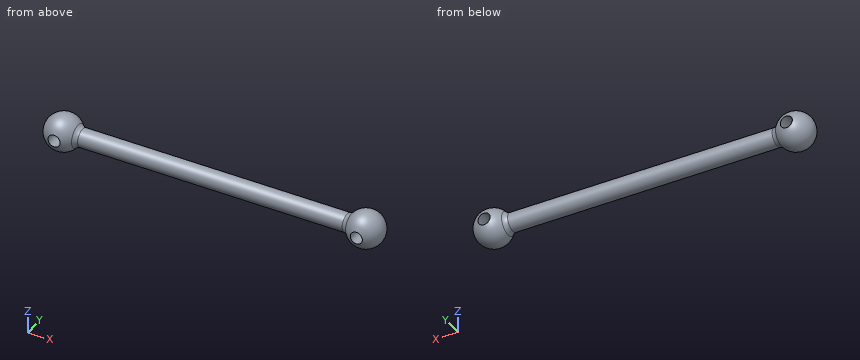
```python
from build123d import *

# Parameters (mm, degrees)
SKETCH1_W          = 23
SKETCH1_H          = 1.5
SKETCH2_R          = 1
CUT_EXTRUDE1_DEPTH = 29.792360098
FILLET1_R          = 1
FILLET2_R          = 1


with BuildPart() as part:
    # Sketch1 → Revolve2 (revolve)
    with BuildSketch(Plane.XY, mode=Mode.PRIVATE) as revolve2_sk:
        with BuildLine():
            Line((23, 1.5), (23, 0))
            Line((23, 0), (28, 0))
            ThreePointArc((28, 0), (25.776457135, 2.897777479), (22.401923789, 1.5))
            Line((22.401923789, 1.5), (23, 1.5))
        make_face()
        with Locations((11.5, 0.75)):
            Rectangle(SKETCH1_W, SKETCH1_H)
    revolve2 = revolve(revolve2_sk.sketch.rotate(Axis((0, 0, 0), (1, 0, 0)), 90), axis=Axis((0, 0, 0), (1, 0, 0)))

    # Sketch2 → Cut-Extrude1 (cut, through all)
    with BuildSketch(Plane(origin=(0, 3, 0), x_dir=(1, 0, 0), z_dir=(0, 1, 0))):
        with Locations(Location((25, 0, 0), (0, 0, 270))):
            Circle(SKETCH2_R)
    cut_extrude1 = extrude(amount=-CUT_EXTRUDE1_DEPTH, mode=Mode.SUBTRACT)

    # Mirror1: Revolve2, Cut-Extrude1 across plane
    add(revolve2.mirror(Plane.ZY))
    add(cut_extrude1.mirror(Plane.ZY), mode=Mode.SUBTRACT)

    # Fillet1
    fillet1_edges = [part.edges().sort_by_distance(p)[0] for p in [
        (22.401923789, 0, -1.5),
    ]]
    fillet(fillet1_edges, radius=FILLET1_R)

    # Fillet2
    fillet2_edges = [part.edges().sort_by_distance(p)[0] for p in [
        (-22.401923789, 0, -1.5),
    ]]
    fillet(fillet2_edges, radius=FILLET2_R)


solid = part.part
```
Work out the finished part from the listing and answer in its coordinate system (mm). Give positions to 0.01 mm unless a question says otherwise; leave off trailing zeros. Order: outer loops, then holes, each group sorted by start corner. A loop starts at its lowest first (then second) coordinate and runs counter-clockwise, first axis right, second up. Notation, with made-up numbers: (46.5, -25) - (75.5, -25) arc R29 ccw to (75.5, 10) - close; hole circle Ø1 at (-32.75, -28). An arc over 180 degrees is marked (long way). One line per item, written item: value. Start each with the question number.
1. Section A-A, the plane x = -25 is taken. Write down the section's boundary in (y, z), then the cut area to 3 significant figures.
2. Section B-B, the plane y = 0 is taken. Count the separate pieces of the cut face and the enclosed holes in it, then the cut area to 3 significant figures.
3. Each of these flat-tipped pins is pushed along its axis until it touches: pin 1 Ø3 at (x, y) = (8.5, 0.5) entering from +Z; pin 2 Ø1.5 at (y, z) = (-2, 0) entering from +X. Where does it stop, or does it pass through?
4. Section D-D, the plane x = -11 is taken. Write down the section's boundary in (y, z).
5. Consider line 1 (X direction, y = 2.2, z = -0.05); line 2 (X direction, y = -0.9, z = 0); line 3 (X direction, y = -0.35, z = -0.2). Determine where each line is inside the solid, lowest interval first.
Filled sheet:
1. outline: (-2.83, -1) arc R3 ccw to (2.83, -1) - close; (-2.83, 1) - (2.83, 1) arc R3 ccw to start
1. area: 16.5 mm²
2. separate pieces: 1
2. enclosed holes: 2
2. area: 183 mm²
3. pin 1: z = 1.5
3. pin 2: x = 27.73
4. outline: circle Ø3 at (0, 0)
5. line 1: -27.04 to -26, -24 to -22.96, 22.96 to 24, 26 to 27.04
5. line 2: -27.86 to -26, -24 to 24, 26 to 27.86
5. line 3: -27.97 to -25.98, -24.02 to 24.02, 25.98 to 27.97
